```python
from build123d import *

# Parameters (mm, degrees)
F0_W      = 133.35
F0_H      = 165.1
F1_DEPTH  = 33.02
F2_W      = 82.55
F2_H      = 73.66
F3_DEPTH  = 33.021
F4_R      = 6.35
F6_D      = 4.826
F7_R      = 7.9375
F7_R_2    = 2.413
F8_DEPTH  = 22.86
F10_D     = 3.175
F10_DEPTH = 12.7
F10_TIP   = 0.9538662327


with BuildPart() as f1:
    # F0 (on Top) → F1 (new body)
    with BuildSketch(Plane.XY):
        Rectangle(F0_W, F0_H)
    extrude(amount=F1_DEPTH)

    # F2 (on face) → F3 (cut, through all)
    with BuildSketch(Plane.XY.offset(33.02)):
        Rectangle(F2_W, F2_H)
    extrude(amount=-F3_DEPTH, mode=Mode.SUBTRACT)

    # F4
    f4_edges = [f1.edges().sort_by_distance(p)[0] for p in [
        (-41.275, 36.83, 16.51),
        (-41.275, -36.83, 16.51),
        (41.275, -36.83, 16.51),
        (41.275, 36.83, 16.51),
    ]]
    fillet(f4_edges, radius=F4_R)

    # F6 (through all)
    with Locations(Plane.XY.offset(33.02)):
        with Locations((-31.75, 52.3875), (31.75, 52.3875), (31.75, -52.3875), (-31.75, -52.3875)):
            Hole(F6_D / 2)

    # F7 (on face) → F8 (cut)
    with BuildSketch(Plane(origin=(0, 0, 0), x_dir=(1, 0, 0), z_dir=(0, 0, -1))):
        with Locations((-31.75, 52.3875)):
            Circle(F7_R)
        with Locations((-31.75, 52.3875)):
            Circle(F7_R_2, mode=Mode.SUBTRACT)
        with Locations((31.75, 52.3875)):
            Circle(F7_R)
        with Locations((31.75, 52.3875)):
            Circle(F7_R_2, mode=Mode.SUBTRACT)
        with Locations((31.75, -52.3875)):
            Circle(F7_R)
        with Locations((31.75, -52.3875)):
            Circle(F7_R_2, mode=Mode.SUBTRACT)
        with Locations((-31.75, -52.3875)):
            Circle(F7_R)
        with Locations((-31.75, -52.3875)):
            Circle(F7_R_2, mode=Mode.SUBTRACT)
    extrude(amount=-F8_DEPTH, mode=Mode.SUBTRACT)

    # F10
    with Locations(Plane(origin=(0, 0, 0), x_dir=(1, 0, 0), z_dir=(0, 0, -1))):
        with Locations((-60.96, 76.835), (60.96, 76.835), (60.96, -76.835), (-60.96, -76.835)):
            Hole(F10_D / 2, depth=F10_DEPTH)
            with Locations((0, 0, -(F10_DEPTH + F10_TIP / 2))):  # 118° drill point
                Cone(0, F10_D / 2, F10_TIP, mode=Mode.SUBTRACT)


solid = f1.part
```
Source: CAD feature listing. Evaluate the final solid. Frame: model axes, mm. A direction names the side the tool comes from. Coordinates: 2 decimals unless noted, no trailing zeros. Write each loop counter-clockwise with the first axis right and the second up, starting at its lowest first coordinate (ties: lowest second). Pieces come first, ordered by that corner, then holes. Notation, with made-up numbers: (8, 48.5) - (64, 48.5) arc R11 ccw to (64, 54.5) - close; hole circle Ø5 at (49.25, 18.25). An arc over 180 degrees is marked (long way). Answer as a JSON object with one key per item and string values.
Q1. Draft query along X for faces 1 (the flat face through (-34, -51, 22.86)), 2 (the flat face through (66.675, -1, 16)), 3 (the flat face through (-1, 38, 33.02)). Return one class per face: released by +X, released by -X, zero draft, split by the parting line, or undercut.
Ans:
{"face 1": "undercut", "face 2": "released by +X", "face 3": "zero draft"}
Q2. Section query B-B, the plane y = -25.5. Output: boundary loops of the cut face in (x, z) (3 decimals).
Ans:
{"outline": "(-66.675, 0) - (-41.275, 0) - (-41.275, 33.02) - (-66.675, 33.02) - close; (41.275, 0) - (66.675, 0) - (66.675, 33.02) - (41.275, 33.02) - close"}
Q3. Section query C-C, the plane x = 15. Output: boundary loops of the cut face in (y, z).
Ans:
{"outline": "(-82.55, 0) - (-36.83, 0) - (-36.83, 33.02) - (-82.55, 33.02) - close; (36.83, 0) - (82.55, 0) - (82.55, 33.02) - (36.83, 33.02) - close"}
Q4. Material intervals for line 1 (Y direction, x = -31.75, z = 11) (3 decimals); line 2 (X direction, y = 29.5, z = 24.5) (3 decimals); line 3 (X direction, y = 53, z = 9.5) (3 decimals), sorted ascending. Write a range as [from, to].
Ans:
{"line 1": "y = [-82.55, -60.325], [-44.45, -36.83], [36.83, 44.45], [60.325, 82.55]", "line 2": "x = [-66.675, -41.275], [41.275, 66.675]", "line 3": "x = [-66.675, -39.664], [-23.836, 23.836], [39.664, 66.675]"}
Q5. Section query A-A, the plane x = -31.75. State how many separate pieces and enclosed holes the cut face has, plus the area to 3 significant figures.
Ans:
{"separate pieces": "4", "enclosed holes": "0", "area": "2,200 mm2"}
Q6. First-contact query: pin 1 Ø8 at (x, y) = (31.5, -54.5) entering from -Z; pin 2 Ø1.9 at (x, y) = (-60.96, -76.835) entering from -Z. Flat tips, straight axial feed; report the tip coordinate or a pass-through.
Ans:
{"pin 1": "stops at z = 22.86", "pin 2": "stops at z = 13.08"}
Q7. Set-up query: faces 4 (the cylindrical face through (-39.365, -35.019, 16.279)), 5 (the flat face through (-1, 38, 0)), 6 (the flat face through (-34, 54, 22.86)). Return all of +Z, -Z, +X, -X, +Y, -Y with unobstructed straight access to the full face (end or side cutting, diameter ignored); none if empty.
Ans:
{"face 4": "+Z, -Z", "face 5": "-Z, +X, -X, +Y, -Y", "face 6": "-Z"}
